```python
from build123d import *

# Parameters (mm, degrees)
F_1_4_CLEARANCE_HOLE1_D = 6.5278
CHAMFER1_SIZE           = 0.762


with BuildPart() as part:
    # Sketch1 → Revolve1 (revolve)
    with BuildSketch(Plane.XY):
        Polygon((7.9375, 0.762), (7.9375, 0), (0, 0), (0, 24.892), (7.9375, 24.892), (7.9375, 24.13), (23.241, 24.13), (23.241, 16.8656), (20.701, 16.8656), (20.701, 14.226799969), (23.241, 14.226799969), (23.241, 8.226800031), (20.701, 8.226800031), (20.701, 5.588), (23.241, 5.588), (23.241, 0.762), align=None)
    revolve(axis=Axis((0, 24.892, 0), (0, -1, 0)))

    # 1/4 Clearance Hole1 (through all)
    with Locations(Plane(origin=(0, 24.892, 0), x_dir=(1, 0, 0), z_dir=(0, 1, 0))):
        with Locations((0, 0)):
            Hole(F_1_4_CLEARANCE_HOLE1_D / 2)

    # Chamfer1
    chamfer1_edges = [part.edges().sort_by_distance(p)[0] for p in [
        (-23.241, 24.13, 0),
        (-23.241, 16.8656, 0),
        (-23.241, 14.226799969, 0),
        (-23.241, 8.226800031, 0),
        (-23.241, 5.588, 0),
        (-23.241, 0.762, 0),
    ]]
    chamfer(chamfer1_edges, length=CHAMFER1_SIZE)


solid = part.part
```
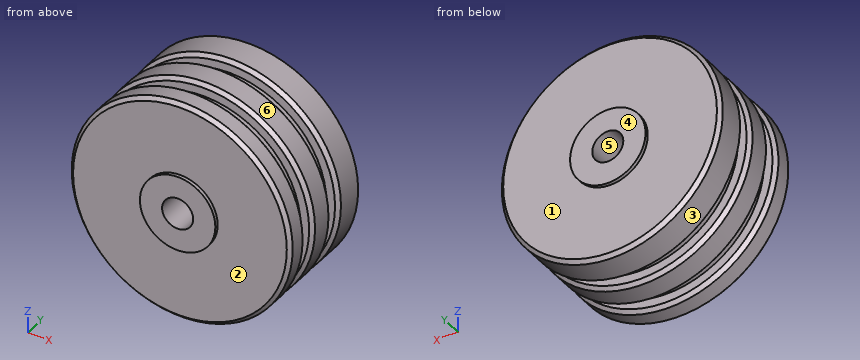
Input: part model. Units: mm. Frame: model coordinates. Face numbers are marked on the shaded views. A direction names the side the tool comes from. Round coordinates to 2 decimals unless told otherwise and drop trailing zeros. Loops run counter-clockwise (first coordinate to the right, second up) from the corner with the lowest first, then second, coordinate; pieces in that order, holes last. Notation, with made-up numbers: (1.25, -18.75) -> (56.25, -18.75) arc R19 cw to (56.25, 15.25) -> close; hole circle Ø6 at (-18, 0.5). An arc over 180 degrees is marked (long way). One line per item, written item: value.
(1) Pin query (flat end, axial travel): pin 1 (1.5 mm diameter, centred on x = 0.5, y = 18, fed in from +Z); pin 2 (6 mm diameter, centred on x = 0, z = 0, fed in from -Y); pin 3 (5 mm diameter, centred on x = 11, y = 18, fed in from -Z); pin 4 (8 mm diameter, centred on x = 9, z = 15, fed in from -Y). Return the tip coordinate at first contact, or that it passes through.
Geometry check:
pin 1: z = 23.24
pin 2: through
pin 3: z = -21.63
pin 4: y = 0.76
(2) Section A-A (y = 12.75). Return the cut outline in (x, z).
Geometry check:
outline: circle Ø46.48 at (0, 0); hole circle Ø6.53 at (0, 0)
(3) Material intervals for line 1 (Y direction, x = 18, z = 13); line 2 (Y direction, x = 17.5, z = 15); line 3 (Z direction, x = 0, y = 13), sorted ascending. Write a range as [from, to].
Geometry check:
line 1: [0.76, 5.59], [8.23, 14.23], [16.87, 24.13]
line 2: [1.33, 5.02], [8.8, 13.66], [17.44, 23.56]
line 3: [-23.24, -3.26], [3.26, 23.24]
(4) Set-up query: the marked faces 1, 2 and 3. Return all of +Z, -Z, +X, -X, +Y, -Y with unobstructed straight access to the full face (end or side cutting, diameter ignored); none if empty.
Geometry check:
face 1: +Y
face 2: -Y
face 3: +Y, -Y
(5) Mould query, pull axis X, two halves, no side actions, for the marked faces 4, 5 and 6. Classes: pulls with the +X half, pulls with the -X half, needs draft (parallel to the pull), parting line crosses it, or undercut.
Geometry check:
face 4: needs draft
face 5: undercut
face 6: parting line crosses it
